Verification items for the finished model (mm, model axes). A direction names the side the tool comes from. Coordinates: 2 decimals unless noted, no trailing zeros. Order: outer loops, then holes, each group sorted by start corner. A loop starts at its lowest first (then second) coordinate and runs counter-clockwise, first axis right, second up. Notation, with made-up numbers: M 38.25,49.25 L 49.25,49.25 A29 ccw 49.25,86.25 Z; hole C 46.5,14.25 d1. An arc over 180 degrees is marked long. Return JSON: item names as keys, results as strings. Group by question number.
Q1. Access from +Z, -Z, +X, -X, +Y, -Y to the whole of each face (thin tool, end or side, straight path). Record for faces 4 (the face through (-15, 12, -5)), 5 (the face through (9, 12, -8)), 6 (the face through (0, 8.5, -5)), 7 (the face through (-11, 5, -3)).
Q2. Thickness scan on probe 1 along Z at (x, y) = (0, 3.5); probe 2 along Y at (x, z) = (-1, -17); probe 3 along X at (y, z) = (22, -11.5). Record the ranges inside material, lowest first.
Q3. Section check B-B, the plane z = -6. Enter the section's corners in (x, y), then the cut area to 3 significant figures.
Q4. Mould release check, pull along Y, two halves, no side actions. Record for faces 1 (the face through (20, 12, -3)), 2 (the face through (-15, 7.5, -3)), 3 (the face through (0, 25, -6)): pulls with the +Y half, pulls with the -Y half, needs draft (parallel to the pull), parting line crosses it, or undercut.
Q5. Go/stop test with flat-tipped pins: pin 1 Ø12 at (y, z) = (13, -15) entering from -X; pin 2 Ø6 at (x, z) = (-2, -8) entering from -Y; pin 3 Ø9 at (x, y) = (-12, 13) entering from -Z; pin 4 Ø2 at (y, z) = (12.5, -11) entering from +X. Record where each tip stops, or that it passes through.
Q6. Section check A-A, the plane y = 22. Enter the section's corners in (x, z), then the cut area to 3 significant figures.
Q7. Section check D-D, the plane x = 6. Enter the section's corners in (y, z).
Q8. Section check C-C, the plane y = 12.5. Enter the section's corners in (x, z).
from build123d import *

# Parameters (mm, degrees)
SKETCH1_R           = 4.5
BOSS_EXTRUDE1_DEPTH = 25
CUT_EXTRUDE1_DEPTH  = 6.5
SKETCH4_W           = 13.2
SKETCH4_H           = 6.5
CUT_EXTRUDE2_DEPTH  = 8.689488223
CUT_EXTRUDE3_DEPTH  = 6


with BuildPart() as part:
    # Sketch1 → Boss-Extrude1 (new body)
    with BuildSketch(Plane(origin=(0, 0, 0), x_dir=(1, 0, 0), z_dir=(0, 1, 0))):
        with BuildLine():
            Line((20, 0), (-20, 0))
            Line((-20, 0), (-20, 5))
            Line((-20, 5), (-9, 5))
            Line((-9, 5), (-9, 11.5))
            ThreePointArc((-9, 11.5), (0, 20.5), (9, 11.5))
            Line((9, 11.5), (9, 5))
            Line((9, 5), (20, 5))
            Line((20, 5), (20, 0))
        make_face()
        with Locations((0, 11.5)):
            Circle(SKETCH1_R, mode=Mode.SUBTRACT)
    extrude(amount=BOSS_EXTRUDE1_DEPTH)

    # Sketch2 → Cut-Extrude1 (cut)
    with BuildSketch(Plane(origin=(0, 15, 0), x_dir=(1, 0, 0), z_dir=(0, 1, 0))):
        Polygon((0, 19.121023553), (-6.6, 15.310511777), (-6.6, 7.689488223), (0, 3.878976447), (6.6, 7.689488223), (6.6, 15.310511777), align=None)
    extrude(amount=-CUT_EXTRUDE1_DEPTH, mode=Mode.SUBTRACT)

    # Sketch4 → Cut-Extrude2 (cut, through all)
    with BuildSketch(Plane(origin=(0, 0, -7.689488223), x_dir=(-1, 0, 0), z_dir=(0, 0, -1))):
        with Locations((0, 11.75)):
            Rectangle(SKETCH4_W, SKETCH4_H)
    extrude(amount=-CUT_EXTRUDE2_DEPTH, mode=Mode.SUBTRACT)

    # Sketch5 → Cut-Extrude3 (cut, through all)
    with BuildSketch(Plane(origin=(0, 0, -5), x_dir=(-1, 0, 0), z_dir=(0, 0, -1))):
        with BuildLine():
            Line((-16, 15), (-13.5, 15))
            ThreePointArc((-13.5, 15), (-11, 12.5), (-13.5, 10))
            Line((-13.5, 10), (-16, 10))
            ThreePointArc((-16, 10), (-18.5, 12.5), (-16, 15))
        make_face()
        with BuildLine():
            Line((13.5, 22.5), (16, 22.5))
            ThreePointArc((16, 22.5), (18.5, 20), (16, 17.5))
            Line((16, 17.5), (13.5, 17.5))
            ThreePointArc((13.5, 17.5), (11, 20), (13.5, 22.5))
        make_face()
        with BuildLine():
            Line((13.5, 7.5), (16, 7.5))
            ThreePointArc((16, 7.5), (18.5, 5), (16, 2.5))
            Line((16, 2.5), (13.5, 2.5))
            ThreePointArc((13.5, 2.5), (11, 5), (13.5, 7.5))
        make_face()
    extrude(amount=-CUT_EXTRUDE3_DEPTH, mode=Mode.SUBTRACT)


solid = part.part
Numbers:
{
 "1": {"face 4": "-Z, -X, +Y, -Y", "face 5": "-Z, +X, +Y, -Y", "face 6": "+Z", "face 7": "+Z, -Z"},
 "2": {"probe 1": "z = -20.5 to -16, -7 to 0", "probe 2": "y = 0 to 8.5, 15 to 25", "probe 3": "x = -9 to -4.5, 4.5 to 9"},
 "3": {"outline": "M -9,0 L 9,0 L 9,25 L -9,25 Z; hole M -6.6,8.5 L 6.6,8.5 L 6.6,15 L -6.6,15 Z", "area": "364 mm2"},
 "4": {"face 1": "needs draft", "face 2": "undercut", "face 3": "pulls with the +Y half"},
 "5": {"pin 1": "stops at x = -9", "pin 2": "stops at y = 0", "pin 3": "stops at z = -16.47", "pin 4": "stops at x = 9"},
 "6": {"outline": "M -20,-5 L -17.5,-5 L -17.5,0 L -20,0 Z; M -12,-5 L -9,-5 L -9,-11.5 A9 ccw 9,-11.5 L 9,-5 L 20,-5 L 20,0 L -12,0 Z; hole C 0,-11.5 d9", "area": "353 mm2"},
 "7": {"outline": "M 0,-18.21 L 25,-18.21 L 25,0 L 15,0 L 15,-15.66 L 8.5,-15.66 L 8.5,0 L 0,0 Z"},
 "8": {"outline": "M -20,-5 L -9,-5 L -9,-11.5 A9 ccw 9,-11.5 L 9,-5 L 11,-5 L 11,0 L 6.6,0 L 6.6,-15.31 L 0,-19.12 L -6.6,-15.31 L -6.6,0 L -20,0 Z; M 18.5,-5 L 20,-5 L 20,0 L 18.5,0 Z"}
}
